Check sheet for the modelled part. Datum: model origin and axes. Units: mm. Give positions to 0.01 mm unless a question says otherwise; leave off trailing zeros. Write each question's results on one line, items separated by ' | '. Start each with the question number.
1. Material ranges on line 1 along Y through (x, z) = (109.5, 8.25); line 2 along X through (y, z) = (-340, 7.75); line 3 along X through (y, z) = (-355, 3.25), recorded low to high.
2. Sectioned sample at A-A on z = 6. Give the number of separate pieces and of enclosed holes in the cut face, and give its area (3 significant figures).
3. Go/stop test with flat-tipped pins: pin 1 (3 mm diameter, centred on y = -563, z = 2.5, fed in from -X); pin 2 (3 mm diameter, centred on x = 474, z = 4.5, fed in from -Y); pin 3 (5 mm diameter, centred on y = -542.5, z = 3.5, fed in from +X). Record where each tip stops, or that it passes through.
```python
from build123d import *

# Parameters (mm, degrees)
EXTRUDE_1_DEPTH     = 10
SKETCH_2_R          = 2.15
CUT_EXTRUDE_1_DEPTH = 10


with BuildPart() as part:
    # 草图1 → 凸台-拉伸1 (new body)
    with BuildSketch(Plane.XY):
        Polygon((0, 0), (0, -535), (20, -535), (20, -555), (40, -555), (40, -575), (460, -575), (460, -555), (480, -555), (480, -535), (500, -535), (500, 0), (480, 0), (480, 20), (460, 20), (460, 40), (40, 40), (40, 20), (20, 20), (20, 0), align=None)
    extrude(amount=EXTRUDE_1_DEPTH)

    # 草图2 → 切除-拉伸1 (cut)
    with BuildSketch(Plane.XY.offset(10)):
        with Locations((64.038059223, -94.038059223)):
            Circle(SKETCH_2_R)
        with Locations((78.180194847, -79.895923599)):
            Circle(SKETCH_2_R)
        with Locations((110, -140)):
            Circle(SKETCH_2_R)
        with Locations((124.142135624, -125.857864376)):
            Circle(SKETCH_2_R)
        with Locations((390, -140)):
            Circle(SKETCH_2_R)
        with Locations((375.857864376, -125.857864376)):
            Circle(SKETCH_2_R)
        with Locations((435.961940777, -94.038059223)):
            Circle(SKETCH_2_R)
        with Locations(Location((421.819805153, -79.895923599, 0), (0, 0, 180))):
            Circle(SKETCH_2_R)
        with Locations((421.819805153, -400.104076401)):
            Circle(SKETCH_2_R)
        with Locations((435.961940777, -385.961940777)):
            Circle(SKETCH_2_R)
        with Locations((375.857864376, -354.142135624)):
            Circle(SKETCH_2_R)
        with Locations((390, -340)):
            Circle(SKETCH_2_R)
        with Locations(Location((124.142135624, -354.142135624, 0), (0, 0, 180))):
            Circle(SKETCH_2_R)
        with Locations(Location((110, -340, 0), (0, 0, 180))):
            Circle(SKETCH_2_R)
        with Locations((78.180194847, -400.104076401)):
            Circle(SKETCH_2_R)
        with Locations((64.038059223, -385.961940777)):
            Circle(SKETCH_2_R)
    extrude(amount=-CUT_EXTRUDE_1_DEPTH, mode=Mode.SUBTRACT)


solid = part.part
```
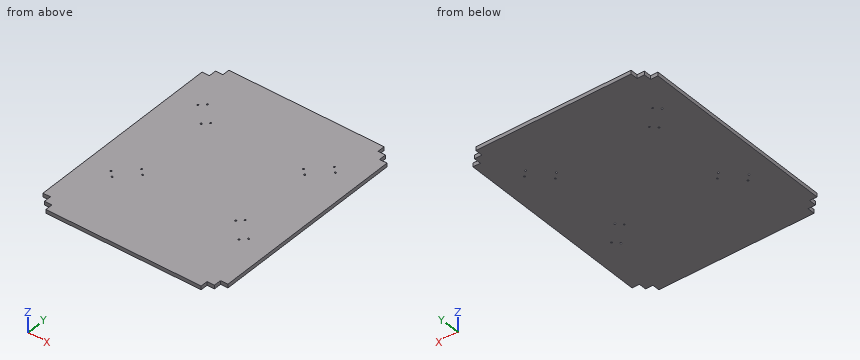
Output values:
1) line 1: -575 to -342.09, -337.91 to -142.09, -137.91 to 40 | line 2: 0 to 107.85, 112.15 to 387.85, 392.15 to 500 | line 3: 0 to 122.17, 126.11 to 373.89, 377.83 to 500
2) separate pieces: 1 | enclosed holes: 16 | area: 302,000 mm2
3) pin 1: x = 40 | pin 2: y = -555 | pin 3: x = 480
